Check sheet for the modelled part. Datum: model origin and axes. Units: mm. Round coordinates to 2 decimals unless told otherwise and drop trailing zeros. Loops run counter-clockwise (first coordinate to the right, second up) from the corner with the lowest first, then second, coordinate; pieces in that order, holes last. Notation, with made-up numbers: M 68,45 L 74,45 A23 ccw 74,55 Z; hole C -1,-11 d6. An arc over 180 degrees is marked long. One line per question, with ' | ' between items. Start each with the question number.
(1) Thickness scan on probe 1 along X at (y, z) = (11.75, 31.2); probe 2 along Z at (x, y) = (-32, 22.75). Record the ranges inside material, lowest first. Write a range as [from, to].
(2) Section check D-D (z = 0). Record the boundary of the cut face in (x, y).
(3) Section check A-A (z = -31.2). Record the boundary of the cut face in (x, y), and give its area (3 significant figures).
(4) Section check C-C (x = 31.2). Record the boundary of the cut face in (y, z), and give its area (3 significant figures).
(5) Section check B-B (y = 20.75). Record the boundary of the cut face in (x, z).
(6) Draft check along X on faces 1 (the face through (39.7, 11.59, -39.77)), 2 (the face through (19, 22.5, 0)), 3 (the face through (1, 12, -41.2)), 4 (the face through (3.945, 11.092, 17.767)). Enter one of: +X half, -X half, draft (parallel to the pull), parting line (faces both ways), or undercut.
(7) Go/stop test with a flat-tipped pin: P1, Ø12, axis at x = -5.5, z = -11, coming from the +Y side. Record where the tip stops, or that it passes through.
Autodesk Inventor part; units mm, degrees
ref_plane "YZ Plane" through (0, 0, 0) normal (1, 0, 0) x (0, 1, 0)
ref_plane "XZ Plane" through (0, 0, 0) normal (0, 1, 0) x (-1, 0, 0)
ref_plane "XY Plane" through (0, 0, 0) normal (0, 0, 1) x (1, 0, 0)
sketch "Boceto1" plane through (0, 0, 0) normal (0, 1, 0) x (-1, 0, 0)
  line L0 (-41.2, 41.2) -> (41.2, 41.2)
  line L1 (41.2, 41.2) -> (41.2, -41.2)
  line L2 (41.2, -41.2) -> (-41.2, -41.2)
  line L3 (-41.2, -41.2) -> (-41.2, 41.2)
  line L4 (-41.2, 41.2) -> (41.2, -41.2) construction
  line L5 (41.2, 41.2) -> (-41.2, -41.2) construction
  circle A0 centre (0, 0) radius 18.2
  dimension "d0" = 82.4
  dimension "d1" = 82.4
  dimension "d2" = 36.4
extrude "Extrusión1" add sketch "Boceto1" along normal blind 22.5
sketch "Boceto2" plane through (0, 22.5, 0) normal (0, 1, 0) x (1, 0, 0)
  circle A0 centre (-31.2, -31.2) radius 2.7
  line L0 (-41.2, 41.2) -> (-41.2, -41.2)
  line L1 (-41.2, -41.2) -> (41.2, -41.2)
  point P0 (0, 0)
  dimension "d5" = 5.4
  dimension "d6" = 10
  dimension "d7" = 10
extrude "Extrusión2" cut sketch "Boceto2" against normal through all
pattern_circular "Patrón circular1" count 4 over 360 about axis through (0, 0, 0) along (0, 1, 0) of "Extrusión2"
fillet "Empalme1" radius 5 4 edges at (-41.2, 11.25, 41.2) (41.2, 11.25, 41.2) (41.2, 11.25, -41.2) (-41.2, 11.25, -41.2)
sketch "Boceto3" plane through (0, 22.5, 0) normal (0, 1, 0) x (1, 0, 0)
  line L0 (-21.2, -21.2) -> (21.2, -21.2)
  line L1 (21.2, -21.2) -> (21.2, 21.2)
  line L2 (21.2, 21.2) -> (-21.2, 21.2)
  line L3 (-21.2, 21.2) -> (-21.2, -21.2)
  line L4 (-21.2, -21.2) -> (21.2, 21.2) construction
  line L5 (21.2, -21.2) -> (-21.2, 21.2) construction
  arc A0 (-36.2, 41.2) -> (-41.2, 36.2) centre (-36.2, 36.2) ccw
  line L6 (-41.2, 36.2) -> (-41.2, -36.2)
  arc A1 (-41.2, -36.2) -> (-36.2, -41.2) centre (-36.2, -36.2) ccw
  line L7 (-36.2, -41.2) -> (36.2, -41.2)
  arc A2 (36.2, -41.2) -> (41.2, -36.2) centre (36.2, -36.2) ccw
  line L8 (41.2, -36.2) -> (41.2, 36.2)
  arc A3 (41.2, 36.2) -> (36.2, 41.2) centre (36.2, 36.2) ccw
  line L9 (36.2, 41.2) -> (-36.2, 41.2)
  circle A4 centre (-31.2, 31.2) radius 2.7
  circle A5 centre (31.2, 31.2) radius 2.7
  circle A6 centre (31.2, -31.2) radius 2.7
  circle A7 centre (-31.2, -31.2) radius 2.7
  circle A8 centre (0, 0) radius 18.2
  dimension "d14" = 42.4
  dimension "d15" = 42.4
extrude "Extrusión3" add sketch "Boceto3" along normal blind 1 contours L9 A3 L8 A2 L7 A1 L6 A0
properties part number "Base"
The answers:
1) probe 1: [-41.2, -33.9], [-28.5, 28.5], [33.9, 41.2] | probe 2: [-41.2, -33.78], [-28.62, 28.62], [33.78, 41.2]
2) outline: M -41.2,0 L -18.2,0 L -18.2,22.5 L -21.2,22.5 L -21.2,23.5 L -41.2,23.5 Z; M 18.2,0 L 41.2,0 L 41.2,23.5 L 21.2,23.5 L 21.2,22.5 L 18.2,22.5 Z
3) outline: M -41.2,0 L -33.9,0 L -33.9,23.5 L -41.2,23.5 Z; M -28.5,0 L 28.5,0 L 28.5,23.5 L -28.5,23.5 Z; M 33.9,0 L 41.2,0 L 41.2,23.5 L 33.9,23.5 Z | area: 1,680 mm²
4) outline: M 0,-41.2 L 23.5,-41.2 L 23.5,-33.9 L 0,-33.9 Z; M 0,-28.5 L 23.5,-28.5 L 23.5,28.5 L 0,28.5 Z; M 0,33.9 L 23.5,33.9 L 23.5,41.2 L 0,41.2 Z | area: 1,680 mm²
5) outline: M -41.2,-36.2 A5 ccw -36.2,-41.2 L 36.2,-41.2 A5 ccw 41.2,-36.2 L 41.2,36.2 A5 ccw 36.2,41.2 L -36.2,41.2 A5 ccw -41.2,36.2 Z; hole C -31.2,-31.2 d5.4; hole C -31.2,31.2 d5.4; hole C 0,0 d36.4; hole C 31.2,-31.2 d5.4; hole C 31.2,31.2 d5.4
6) face 1: +X half | face 2: undercut | face 3: draft | face 4: undercut
7) P1: y = 22.5
